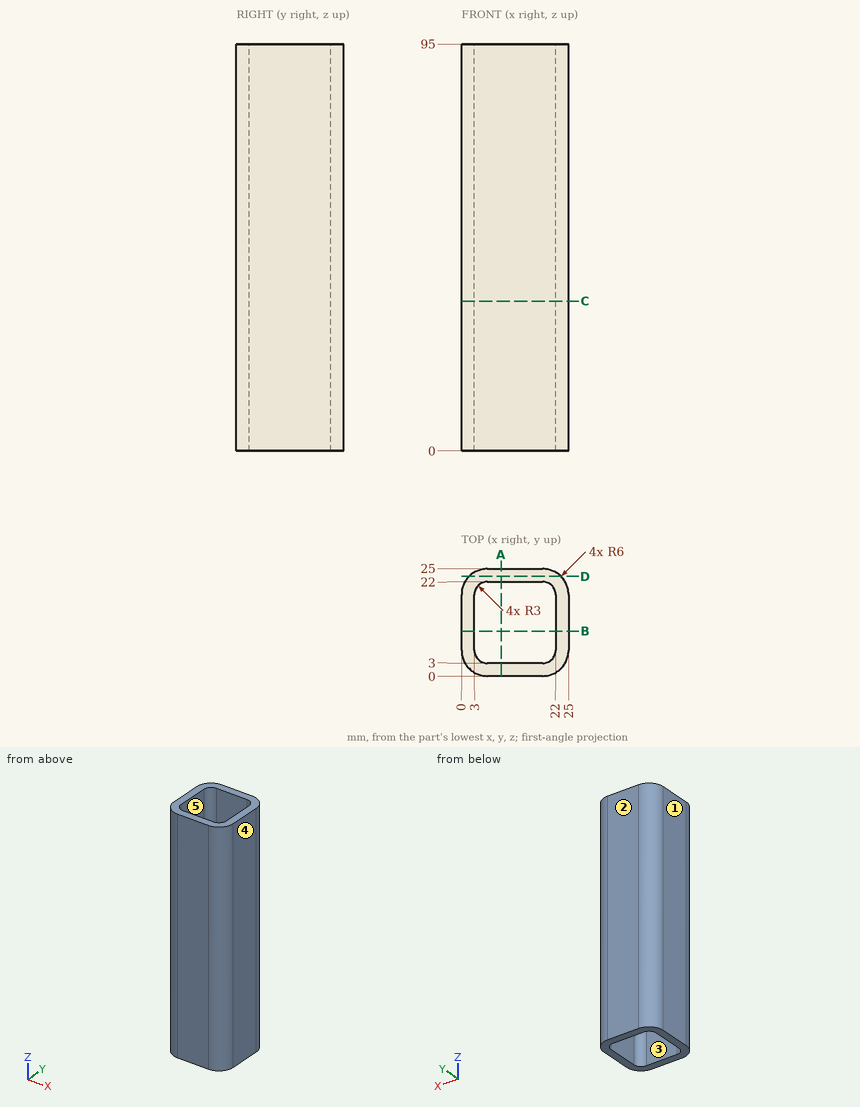
The drawing under review shows one solid part. Ordinate dimensions are in mm from its lowest x, y, z. A direction names the side the tool comes from. Give positions to 0.01 mm unless a question says otherwise; leave off trailing zeros. Write each loop counter-clockwise with the first axis right and the second up, starting at its lowest first coordinate (ties: lowest second). Pieces come first, ordered by that corner, then holes. Notation, with made-up numbers: (76, 27) -> (96, 27) arc R7 ccw to (96, 33) -> close; hole circle Ø2 at (-30, 32). An arc over 180 degrees is marked (long way). Answer in a Markdown table with one row per item.
(1) Consider section D-D (y = 23.25). State the section outline as (x, z) points, then the cut area to 3 significant figures.
Results:
| item | result |
|---|---|
| outline | (1.76, 0) -> (23.24, 0) -> (23.24, 95) -> (1.76, 95) -> close |
| area | 2,040 mm2 |
(2) For the marked faces 4 and 5, list the 3-axis set-ups (+Z, -Z, +X, -X, +Y, -Y) from which the entire face can be reached by the end or side of a thin tool; tool diameter is ignored.
Results:
| item | result |
|---|---|
| face 4 | +Z, -Z, +X, +Y, -Y |
| face 5 | +Z, -Z |
(3) Mouldability with a two-part tool opening along Y and no side actions: class the marked faces 1, 2 and 3 as +Y half, -Y half, draft (parallel to the pull), parting line (faces both ways), or undercut.
Results:
| item | result |
|---|---|
| face 1 | draft |
| face 2 | +Y half |
| face 3 | undercut |
(4) To check wall thickness, follow probe 1 along X at (y, z) = (13.5, 4); probe 2 along Y at (x, z) = (5, 58). State the ranges of each line that lie inside material, in increasing order.
Results:
| item | result |
|---|---|
| probe 1 | 0 to 3, 22 to 25 |
| probe 2 | 0.08 to 3.17, 21.83 to 24.92 |
(5) Consider section A-A (x = 9.25). State the section outline as (y, z) points, then the cut area to 3 significant figures.
Results:
| item | result |
|---|---|
| outline | (0, 0) -> (3, 0) -> (3, 95) -> (0, 95) -> close; (22, 0) -> (25, 0) -> (25, 95) -> (22, 95) -> close |
| area | 570 mm2 |
(6) Consider section C-C (z = 35). State the section outline as (x, y) points.
Results:
| item | result |
|---|---|
| outline | (0, 6) arc R6 ccw to (6, 0) -> (19, 0) arc R6 ccw to (25, 6) -> (25, 19) arc R6 ccw to (19, 25) -> (6, 25) arc R6 ccw to (0, 19) -> close; hole (3, 6) arc R3 ccw to (6, 3) -> (19, 3) arc R3 ccw to (22, 6) -> (22, 19) arc R3 ccw to (19, 22) -> (6, 22) arc R3 ccw to (3, 19) -> close |
